Verification items for the finished model (mm, model axes). Give positions to 0.01 mm unless a question says otherwise; leave off trailing zeros. Write each loop counter-clockwise with the first axis right and the second up, starting at its lowest first coordinate (ties: lowest second). Pieces come first, ordered by that corner, then holes. Notation, with made-up numbers: (-14, -33.75) - (2, -33.75) arc R20 cw to (2, -4.75) - close; hole circle Ø8 at (64.25, -21). An arc over 180 degrees is marked (long way). Put each result on its own line as item: value.
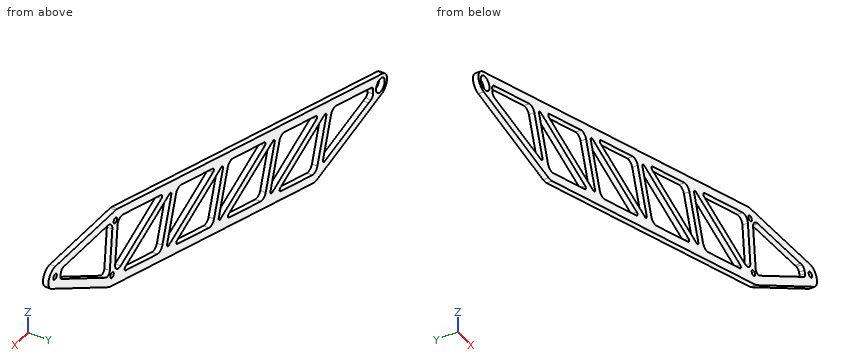
from build123d import *

# Parameters (mm, degrees)
BOSS_EXTRUDE1_DEPTH      = 3.175
BOSS_EXTRUDE1_DEPTH_BACK = 3.175
SKETCH2_R                = 8.334375
SKETCH2_R_2              = 3.302
CUT_EXTRUDE1_DEPTH       = 663.832858032
RIGHT_ANGLES_R           = 7.62
FILLET9_R                = 9.398
FILLET10_R               = 7.62
FILLET11_R               = 5.08
FILLET13_R               = 5.08
FILLET14_R               = 2.54


with BuildPart() as part:
    # Sketch2 → Boss-Extrude1 (new, two sides: drawn at the far end of the back side and taken through both)
    with BuildSketch(Plane(origin=(0, 0, 0), x_dir=(1, 0, 0), z_dir=(0, 1, 0)).offset(-BOSS_EXTRUDE1_DEPTH_BACK)):
        with BuildLine():
            Line((-3.965619751, -12.064984873), (504.134113458, -179.071438566))
            ThreePointArc((504.134113458, -179.071438566), (505.781320473, -179.493044996), (507.470083881, -179.690835496))
            Line((507.470083881, -179.690835496), (623.002452599, -185.425831444))
            ThreePointArc((623.002452599, -185.425831444), (635.721308663, -176.632603773), (630.519585141, -162.071277432))
            Line((630.519585141, -162.071277432), (521.293179876, -91.566789023))
            ThreePointArc((521.293179876, -91.566789023), (519.876879037, -90.77588958), (518.371316412, -90.171976358))
            Line((518.371316412, -90.171976358), (128.279552471, 38.046634777))
            ThreePointArc((128.279552471, 38.046634777), (125.021779391, 38.661908304), (121.715767729, 38.413043176))
            Line((121.715767729, 38.413043176), (-2.59816499, 12.431393272))
            ThreePointArc((-2.59816499, 12.431393272), (-12.6802584, 0.707846671), (-3.965619751, -12.064984873))
        make_face()
        with Locations(Location((0, 0, 0), (0, 0, 270))):
            Circle(SKETCH2_R, mode=Mode.SUBTRACT)
        with Locations(Location((623.632101926, -172.741449641, 0), (0, 0, 270))):
            Circle(SKETCH2_R_2, mode=Mode.SUBTRACT)
        with Locations(Location((508.099733209, -167.006453693, 0), (0, 0, 270))):
            Circle(SKETCH2_R_2, mode=Mode.SUBTRACT)
        with Locations(Location((514.405696661, -102.236961232, 0), (0, 0, 270))):
            Circle(SKETCH2_R_2, mode=Mode.SUBTRACT)
    extrude(amount=BOSS_EXTRUDE1_DEPTH + BOSS_EXTRUDE1_DEPTH_BACK)

    # Sketch4 → Cut-Extrude1 (cut, through all)
    with BuildSketch(Plane(origin=(0, 3.175, 0), x_dir=(1, 0, 0), z_dir=(0, 1, 0))):
        Polygon((123.173594128, 29.030153456), (101.759247472, -36.120764859), (197.883708709, 4.473810527), align=None)
        Polygon((212.569250905, -0.353155839), (116.444789668, -40.947731225), (191.154904249, -65.504074154), align=None)
        Polygon((222.221238803, -3.52565164), (200.806892147, -68.676569955), (296.931353384, -28.08199457), align=None)
        Polygon((311.61689558, -32.908960935), (215.492434343, -73.503536321), (290.202548924, -98.059879251), align=None)
        Polygon((321.268883479, -36.081456736), (299.854536823, -101.232375051), (395.97899806, -60.637799666), align=None)
        Polygon((410.664540256, -65.464766032), (314.540079019, -106.059341417), (389.2501936, -130.615684347), align=None)
        Polygon((519.484855658, -102.492310656), (512.932796085, -169.789493129), (604.57066912, -174.338372689), (611.078066813, -174.661398174), (614.555007617, -163.859087404), (609.080948645, -160.325640282), align=None)
        Polygon((509.712184931, -98.020571128), (413.587723694, -138.615146514), (502.901744402, -167.971622986), align=None)
        Polygon((420.316528154, -68.637261833), (398.902181498, -133.788180148), (495.026642735, -93.193604762), align=None)
        Polygon((22.677662652, 7.33452053), (111.445751733, 25.887078258), (92.107259573, -32.948269058), (21.720444319, -9.812944172), (13.482358668, -7.105181542), (14.189389884, 5.560468929), align=None)
    extrude(amount=-CUT_EXTRUDE1_DEPTH, mode=Mode.SUBTRACT)

    # right angles
    right_angles_edges = [part.edges().sort_by_distance(p)[0] for p in [
        (389.2501936, 0, 130.615684347),
        (92.107259573, 0, 32.948269058),
        (502.901744402, 0, 167.971622986),
        (222.221238803, 0, 3.52565164),
        (191.154904249, 0, 65.504074154),
        (321.268883479, 0, 36.081456736),
        (290.202548924, 0, 98.059879251),
        (420.316528154, 0, 68.637261833),
        (123.173594128, 0, -29.030153456),
    ]]
    fillet(right_angles_edges, radius=RIGHT_ANGLES_R)

    # Fillet9
    fillet9_edges = [part.edges().sort_by_distance(p)[0] for p in [
        (512.932796085, 0, 169.789493129),
    ]]
    fillet(fillet9_edges, radius=FILLET9_R)

    # Fillet10
    fillet10_edges = [part.edges().sort_by_distance(p)[0] for p in [
        (509.712184931, 0, 98.020571128),
    ]]
    fillet(fillet10_edges, radius=FILLET10_R)

    # Fillet11
    fillet11_edges = [part.edges().sort_by_distance(p)[0] for p in [
        (519.484855658, 0, 102.492310656),
    ]]
    fillet(fillet11_edges, radius=FILLET11_R)

    # Fillet13
    fillet13_edges = [part.edges().sort_by_distance(p)[0] for p in [
        (614.555007617, 0, 163.859087404),
        (611.078066813, 0, 174.661398174),
        (13.482358668, 0, 7.105181542),
        (14.189389884, 0, -5.560468929),
    ]]
    fillet(fillet13_edges, radius=FILLET13_R)

    # Fillet14
    fillet14_edges = [part.edges().sort_by_distance(p)[0] for p in [
        (410.664540256, 0, 65.464766032),
        (314.540079019, 0, 106.059341417),
        (111.445751733, 0, -25.887078258),
        (413.587723694, 0, 138.615146514),
        (296.931353384, 0, 28.08199457),
        (200.806892147, 0, 68.676569955),
        (212.569250905, 0, 0.353155839),
        (116.444789668, 0, 40.947731225),
        (395.97899806, 0, 60.637799666),
        (299.854536823, 0, 101.232375051),
        (311.61689558, 0, 32.908960935),
        (215.492434343, 0, 73.503536321),
        (495.026642735, 0, 93.193604762),
        (398.902181498, 0, 133.788180148),
        (197.883708709, 0, -4.473810527),
        (101.759247472, 0, 36.120764859),
    ]]
    fillet(fillet14_edges, radius=FILLET14_R)


solid = part.part
Q1. Go/stop test with a flat-tipped pin: pin 1 Ø6 at (x, z) = (623.63, 172.74) entering from -Y. Record where the tip stops, or that it passes through.
Answers follow:
pin 1: passes through
Q2. Scan lines: line 1 along Z through (x, y) = (322.5, -1); line 2 along Z through (x, y) = (337, -1); line 3 along Z through (x, y) = (524, -1.75). Record each from-to range of solid material in increasing order.
Answers follow:
line 1: z = 25.79 to 39, 91.67 to 102.7, 108.68 to 119.37
line 2: z = 30.56 to 41.25, 85.55 to 96.57, 113.44 to 124.14
line 3: z = 93.31 to 106.21, 170.34 to 180.51
Q3. Section check A-A, the plane z = 147. Record the cut outline in (x, y) (3 decimals).
Answers follow:
outline: (406.56, -3.175) - (439.098, -3.175) - (439.098, 3.175) - (406.56, 3.175) - close; (504.944, -3.175) - (515.152, -3.175) - (515.152, 3.175) - (504.944, 3.175) - close; (588.437, -3.175) - (607.171, -3.175) - (607.171, 3.175) - (588.437, 3.175) - close
Q4. Section check B-B, the plane x = 267. Record the cut outline in (y, z) (3 decimals), plus the area to 3 significant figures.
Answers follow:
outline: (-3.175, 7.549) - (3.175, 7.549) - (3.175, 18.244) - (-3.175, 18.244) - close; (-3.175, 40.722) - (3.175, 40.722) - (3.175, 51.751) - (-3.175, 51.751) - close; (-3.175, 90.433) - (3.175, 90.433) - (3.175, 101.128) - (-3.175, 101.128) - close
area: 206 mm2
Q5. Section check C-C, the plane y = 1.5. Give the number of separate pieces and of enclosed holes in the cut face, plus the area to 3 significant figures.
Answers follow:
separate pieces: 1
enclosed holes: 14
area: 21,800 mm2
